```python
from build123d import *

# Parameters (mm, degrees)
EXTRUDE_1_DEPTH             = 10
CUT_EXTRUDE_1_DEPTH         = 11
CUT_EXTRUDE_2_DEPTH         = 11
HOLE_WIZARD_3_6_3_6_1_D     = 3.6
HOLE_WIZARD_3_6_3_6_1_DEPTH = 10
FILLET_1_R                  = 2


with BuildPart() as part:
    # 草图1 → 凸台-拉伸1 (new body)
    with BuildSketch(Plane.XY.offset(10)):
        with BuildLine():
            Line((-457.29725976, 133), (-442.70274024, 133))
            ThreePointArc((-442.70274024, 133), (-450, 168.5), (-457.29725976, 133))
        make_face()
    extrude(amount=-EXTRUDE_1_DEPTH)

    # 草图2 → 切除-拉伸1 (cut, through all)
    with BuildSketch(Plane(origin=(0, 0, 0), x_dir=(-1, 0, 0), z_dir=(0, 0, -1))):
        with BuildLine():
            Line((431.781056569, 146.787508713), (435.227883705, 147.395277335))
            ThreePointArc((435.227883705, 147.395277335), (437.009618943, 157.5), (444.86969785, 164.095389312))
            Line((444.86969785, 164.095389312), (443.672627348, 167.384313485))
            ThreePointArc((443.672627348, 167.384313485), (433.97853003, 159.25), (431.781056569, 146.787508713))
        make_face()
    extrude(amount=-CUT_EXTRUDE_1_DEPTH, mode=Mode.SUBTRACT)

    # 草图3 → 切除-拉伸2 (cut, through all)
    with BuildSketch(Plane(origin=(0, 0, 0), x_dir=(-1, 0, 0), z_dir=(0, 0, -1))):
        with BuildLine():
            Line((456.327372652, 167.384313485), (455.13030215, 164.095389312))
            ThreePointArc((455.13030215, 164.095389312), (462.990381057, 157.5), (464.772116295, 147.395277335))
            Line((464.772116295, 147.395277335), (468.218943431, 146.787508713))
            ThreePointArc((468.218943431, 146.787508713), (466.02146997, 159.25), (456.327372652, 167.384313485))
        make_face()
    extrude(amount=-CUT_EXTRUDE_2_DEPTH, mode=Mode.SUBTRACT)

    # Ø3.6 (3.6) 直径孔1
    with Locations(Plane(origin=(0, 0, 0), x_dir=(-1, 0, 0), z_dir=(0, 0, -1))):
        with Locations((437.009618943, 142.5), (450, 165), (462.990381057, 142.5)):
            Hole(HOLE_WIZARD_3_6_3_6_1_D / 2, depth=HOLE_WIZARD_3_6_3_6_1_DEPTH)

    # 草图6 → M12 六角头螺栓的柱形沉头孔1 (revolve, cut)
    with BuildSketch(Plane(origin=(-450, 150, 10), x_dir=(0, -1, 0), z_dir=(1, 0, 0))):
        Polygon((0, 0), (0, 10), (10, 10), (7.5, 5), (7.5, 4), (11.25, 4), (11.25, 0), align=None)
    revolve(axis=Axis((-450, 150, 16.35), (0, 0, -1)), mode=Mode.SUBTRACT)

    # 圆角1
    fillet_1_edges = [part.edges().sort_by_distance(p)[0] for p in [
        (-444.86969785, 164.095389312, 5),
        (-435.227883705, 147.395277335, 5),
        (-464.772116295, 147.395277335, 5),
        (-455.13030215, 164.095389312, 5),
    ]]
    fillet(fillet_1_edges, radius=FILLET_1_R)


solid = part.part
```
Can you work these out from the model? Positions are in its coordinate system, mm. A direction names the side the tool comes from. Coordinates: 2 decimals unless noted, no trailing zeros. Write each loop counter-clockwise with the first axis right and the second up, starting at its lowest first coordinate (ties: lowest second). Pieces come first, ordered by that corner, then holes. Notation, with made-up numbers: (1.25, 1) - (36.25, 1) arc R14 ccw to (36.25, 7) - close; hole circle Ø3 at (8, 44.5). An arc over 180 degrees is marked (long way). Return JSON: item names as keys, results as strings.
Q1. Thinking about a two-plate mould opening in Y: for faces 1 (the flat face through (-450, 139, 0)), 2 (the cylindrical face through (-449.9, 168.5, 5.1)), 3 (the flat face through (-443.953, 166.613, 4.93)), 4 (the flat face through (-450, 133, 5)), which applies, +Y half, -Y half, draft (parallel to the pull), parting line (faces both ways), or undercut?
Computed values:
{"face 1": "draft", "face 2": "+Y half", "face 3": "undercut", "face 4": "-Y half"}
Q2. If we section it at B-B (x = -462): Please give me the cut outline in (y, z).
Computed values:
{"outline": "(135.92, 0) - (141, 0) - (141, 10) - (135.92, 10) - close; (144, 0) - (159, 0) - (159, 10) - (144, 10) - close"}
Q3. On a 3-axis mill with a long thin cutter (end or side, diameter ignored), from which of +Z, -Z, +X, -X, +Y, -Y can I reach the whole of each face in a straight line? I mean faces 5 (the flat face through (-442.7, 152.3, 6)), 6 (the conical face through (-457.557, 150.992, 4.757)), 7 (the flat face through (-456.055, 166.635, 4.93)). Say none if no direction works.
Computed values:
{"face 5": "+Z", "face 6": "-Z", "face 7": "+Z, -Z, -X"}
Q4. If we section it at C-C (z = 0.75): Count the separate pieces of the cut face and the enclosed holes in it, then the cut area to 3 significant figures.
Computed values:
{"separate pieces": "1", "enclosed holes": "4", "area": "578 mm2"}
Q5. If we section it at A-A (y = 150): Please give me the cut outline in (x, z), then the cut area to 4 significant figures.
Computed values:
{"outline": "(-465, 0) - (-460, 0) - (-457.5, 5) - (-457.5, 6) - (-461.25, 6) - (-461.25, 10) - (-465, 10) - close; (-442.5, 5) - (-440, 0) - (-435, 0) - (-435, 10) - (-438.75, 10) - (-438.75, 6) - (-442.5, 6) - close", "area": "107.5 mm2"}
Q6. I'm going to push flat-ended pins straight in: pin 1 Ø3 at (x, y) = (-450, 165) entering from +Z; pin 2 Ø6 at (y, z) = (155.5, 8) entering from -X; pin 3 Ø6 at (x, z) = (-441.5, 1) entering from +Y; pin 4 Ø6 at (x, z) = (-441.5, 3.5) entering from -Y. Where does each tip first touch, or does it pass through?
Computed values:
{"pin 1": "passes through", "pin 2": "stops at x = -464.79", "pin 3": "stops at y = 167.66", "pin 4": "stops at y = 133"}
Q7. Please list where these lines run through material, in increasing order: L1, parallel to Y at x = -450, z = 5; L2, parallel to Y at x = -450, z = 7.55; L3, parallel to X at y = 144, z = 2.75. Write a range as from..to.
Computed values:
{"L1": "y = 133..142.5, 157.5..163.2, 166.8..168.5", "L2": "y = 133..138.75, 161.25..163.2, 166.8..168.5", "L3": "x = -467.5..-463.99, -462..-456.2, -443.8..-438, -436.01..-432.5"}
